Build history of the part. All positions in model axes, mm. Face numbers are marked on the shaded views. A direction names the side the tool comes from. Coordinates: 2 decimals unless noted, no trailing zeros. Loops run counter-clockwise (first coordinate to the right, second up) from the corner with the lowest first, then second, coordinate; pieces in that order, holes last.
Item 1: Cut at A-A (z = 6.5). List the corners of the cut face in (x, y) (3 decimals).
Item 2: Flat gauge pins, fed straight in: pin 1 (15 mm diameter, centred on x = 90.5, y = 8, fed in from -Z); pin 2 (5 mm diameter, centred on y = 37, z = 5, fed in from +X) (3 decimals); pin 3 (12 mm diameter, centred on y = 19.5, z = 33.5, fed in from +X); pin 4 (19 mm diameter, centred on y = -17, z = 15, fed in from -X) (3 decimals). Where does each tip first touch, or does it go through?
Item 3: Drill centre lines: line 1 along Z through (x, y) = (25, 41) (3 decimals); line 2 along Y through (x, z) = (8, 17); line 3 along Y through (x, z) = (25.5, 36). Where is each one in solid material? Low to high.
Item 4: Cut at B-B (x = 82). List the corners of the cut face in (y, z).
Item 5: 3-axis set-ups, long thin cutter, end or side, ignore diameter. For the marked faces 1, 2, 3, 4 and 5: which of +Z, -Z, +X, -X, +Y, -Y reach the whole face in a straight line?
from build123d import *

# Parameters (mm, degrees)
F1_DEPTH = 63.5
F2_DEPTH = 25.4
F0_W     = 25.4
F0_H     = 19.05
F3_DEPTH = 25.4
F4_DEPTH = 7.9375
F5_DEPTH = 25.4
F7_R     = 12.7


with BuildPart() as f1:
    # F0 (on Front) → F1 (new body, symmetric)
    with BuildSketch(Plane.XZ):
        Polygon((22.225, 9.525), (-41.275, 9.525), (-41.275, -9.525), (41.275, -9.525), (41.275, 9.525), align=None)
    extrude(amount=F1_DEPTH, both=True)

    # F0 (on Front) → F2 (join, symmetric)
    with BuildSketch(Plane.XZ):
        with BuildLine():
            Line((22.225, 27.0002), (22.225, 9.525))
            Line((22.225, 9.525), (41.275, 9.525))
            Line((41.275, 9.525), (41.275, 27.0002))
            ThreePointArc((41.275, 27.0002), (45.92468, 38.22552), (57.15, 42.8752))
            Line((57.15, 42.8752), (60.325, 42.8752))
            Line((60.325, 42.8752), (60.325, 61.9252))
            Line((60.325, 61.9252), (57.15, 61.9252))
            add(Edge.make_bspline(
                [(51.038245, 61.386274), (53.028106, 61.581124), (55.064944, 61.76099), (57.15, 61.9252)],
                knots=[108.753327, 108.753327, 108.753327, 108.753327, 111.504536, 111.504536, 111.504536, 111.504536], degree=3))
            ThreePointArc((51.038245, 61.386274), (30.380534, 49.431234), (22.225, 27.0002))
        make_face()
    extrude(amount=F2_DEPTH, both=True)

    # F0 (on Front) → F3 (join, symmetric)
    with BuildSketch(Plane.XZ):
        with Locations((73.025, 52.4002)):
            Rectangle(F0_W, F0_H)
    extrude(amount=F3_DEPTH, both=True)

    # F0 (on Front) → F4 (join, symmetric)
    with BuildSketch(Plane.XZ):
        with BuildLine():
            add(Edge.make_bspline(
                [(-41.275, 9.525), (-32.871462, 22.567717), (-27.619523, 53.683983), (51.038245, 61.386274)],
                knots=[0, 0, 0, 0, 108.753327, 108.753327, 108.753327, 108.753327], degree=3))
            Line((-41.275, 9.525), (22.225, 9.525))
            Line((22.225, 9.525), (22.225, 27.0002))
            ThreePointArc((22.225, 27.0002), (30.380534, 49.431234), (51.038245, 61.386274))
        make_face()
    extrude(amount=F4_DEPTH, both=True)

    # F0 (on Front) → F5 (join, symmetric)
    with BuildSketch(Plane.XZ):
        with Locations((73.025, 52.4002)):
            Rectangle(F0_W, F0_H)
    extrude(amount=F5_DEPTH, both=True)

    # F0 (on Front) → F6 (revolve)
    with BuildSketch(Plane.XZ):
        Polygon((85.725, 66.6877), (85.725, 61.9252), (85.725, 42.8752), (85.725, 38.1127), (111.125, 38.1127), (111.125, 66.6877), align=None)
    revolve(axis=Axis((85.725, 0, 52.4002), (0, 0, -1)))

    # F7
    f7_edges = [f1.edges().sort_by_distance(p)[0] for p in [
        (-41.275, -63.5, 0),
        (41.275, -63.5, 0),
        (41.275, 63.5, 0),
        (-41.275, 63.5, 0),
    ]]
    fillet(f7_edges, radius=F7_R)


solid = f1.part
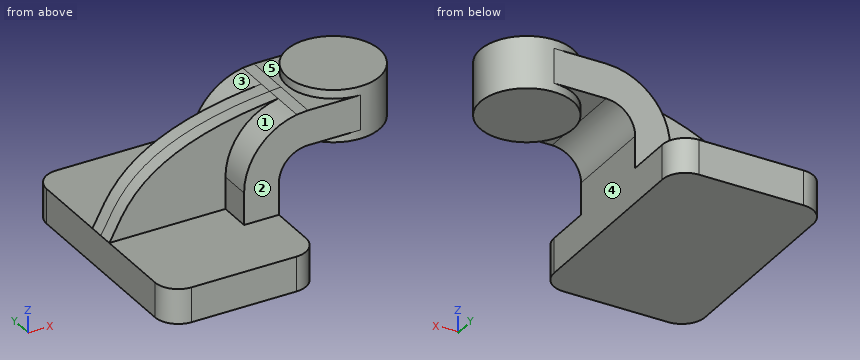
Filled sheet:
1. outline: (-41.275, -50.8) arc R12.7 ccw to (-28.575, -63.5) - (28.575, -63.5) arc R12.7 ccw to (41.275, -50.8) - (41.275, 50.8) arc R12.7 ccw to (28.575, 63.5) - (-28.575, 63.5) arc R12.7 ccw to (-41.275, 50.8) - close
2. pin 1: stops at z = 38.11
2. pin 2: stops at x = 41.275
2. pin 3: stops at x = 105.72
2. pin 4: stops at x = -41.275
3. line 1: z = -9.525 to 9.525
3. line 2: y = -7.94 to 7.94
3. line 3: y = -25.4 to 25.4
4. outline: (-25.4, 42.88) - (-25.13, 42.88) - (-25.13, 38.11) - (25.13, 38.11) - (25.13, 42.88) - (25.4, 42.88) - (25.4, 61.93) - (25.13, 61.93) - (25.13, 66.69) - (-25.13, 66.69) - (-25.13, 61.93) - (-25.4, 61.93) - close
5. face 1: +Z, -X, -Y
5. face 2: +Z, +X, -X, -Y
5. face 3: +Z, -X, +Y
5. face 4: -Z, +X, +Y, -Y
5. face 5: +Z, -X
